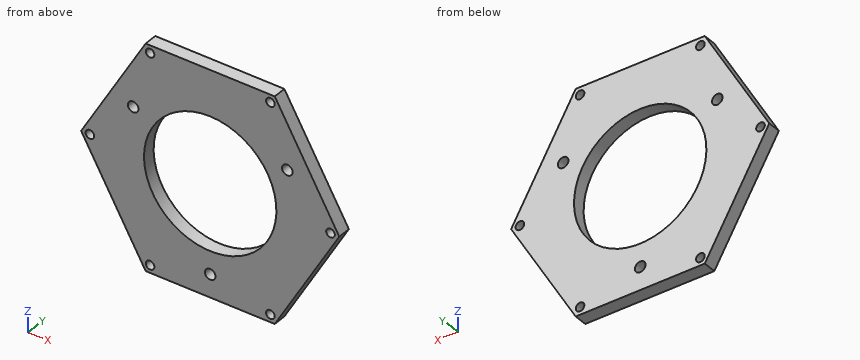
```python
from build123d import *

# Parameters (mm, degrees)
BOSS_EXTRUDE1_DEPTH = 4
SKETCH3_R           = 20
CUT_EXTRUDE1_DEPTH  = 4
SKETCH4_R           = 1.6
SKETCH4_R_2         = 1.3
CUT_EXTRUDE2_DEPTH  = 4


with BuildPart() as part:
    # Sketch2 → Boss-Extrude1 (new body)
    with BuildSketch(Plane(origin=(0, 0, 0), x_dir=(1, 0, 0), z_dir=(0, 1, 0))):
        Polygon((1.572650536, 74.401195204), (-37.427349464, 74.401195204), (-56.927349464, 40.626204456), (-37.427349464, 6.851213708), (1.572650536, 6.851213708), (21.072650536, 40.626204456), align=None)
    extrude(amount=-BOSS_EXTRUDE1_DEPTH)

    # Sketch3 → Cut-Extrude1 (cut)
    with BuildSketch(Plane(origin=(0, 0, 0), x_dir=(1, 0, 0), z_dir=(0, 1, 0))):
        with Locations(Location((-17.927354806, 40.626195204, 0), (0, 0, 270))):
            Circle(SKETCH3_R)
    extrude(amount=-CUT_EXTRUDE1_DEPTH, mode=Mode.SUBTRACT)

    # Sketch4 → Cut-Extrude2 (cut)
    with BuildSketch(Plane(origin=(0, 0, 0), x_dir=(1, 0, 0), z_dir=(0, 1, 0))):
        with Locations(Location((5.360065631, 27.181209082, 0), (0, 0, 270))):
            Circle(SKETCH4_R)
        with Locations(Location((0.244744901, 9.15121368, 0), (0, 0, 270))):
            Circle(SKETCH4_R_2)
        with Locations(Location((-36.099443845, 9.151213708, 0), (0, 0, 270))):
            Circle(SKETCH4_R_2)
        with Locations(Location((-41.214764559, 27.181190577, 0), (0, 0, 270))):
            Circle(SKETCH4_R)
        with Locations(Location((-17.927365489, 67.516185951, 0), (0, 0, 270))):
            Circle(SKETCH4_R)
        with Locations(Location((18.416839298, 40.626204456, 0), (0, 0, 270))):
            Circle(SKETCH4_R_2)
        with Locations(Location((0.244744917, 72.101195204, 0), (0, 0, 270))):
            Circle(SKETCH4_R_2)
        with Locations(Location((-54.271538226, 40.626204456, 0), (0, 0, 270))):
            Circle(SKETCH4_R_2)
        with Locations(Location((-36.099443845, 72.101195204, 0), (0, 0, 270))):
            Circle(SKETCH4_R_2)
    extrude(amount=-CUT_EXTRUDE2_DEPTH, mode=Mode.SUBTRACT)


solid = part.part
```
Read the model definition and answer for the solid it produces. Units are mm, in the model's axes. Round coordinates to 2 decimals unless told otherwise and drop trailing zeros. Write each loop counter-clockwise with the first axis right and the second up, starting at its lowest first coordinate (ties: lowest second). Pieces come first, ordered by that corner, then holes. Notation, with made-up numbers: (-20, -36.5) - (-8, -36.5) arc R19 ccw to (-8, -24.5) - close; hole circle Ø7 at (60, 63). An arc over 180 degrees is marked (long way). One line per item, written item: value.
Q1. Straight lines are drawn through the part: line 1 (X direction, y = -2.5, z = -28.5); line 2 (Z direction, x = -19, y = -1.35); line 3 (Z direction, x = 18, y = -0.8). For each, find the intervals that lie inside material, in ascending order. Write a range as from..to.
The answers:
line 1: x = -49.93..-42.12, -40.31..-33.83, -2.02..4.45, 6.27..14.07
line 2: z = -74.4..-68.7, -66.33..-60.6, -20.65..-6.85
line 3: z = -45.95..-41.86, -39.39..-35.3
Q2. Find section C-C (y = -3.4). Count the separate pieces of the cut face and the enclosed holes in it, and give its area (3 significant figures).
The answers:
separate pieces: 1
enclosed holes: 10
area: 2,640 mm2
Q3. Find section A-A (z = -24). Determine the outline of the cut face in (x, y), and give its area (3 significant figures).
The answers:
outline: (-47.33, -4) - (-29.04, -4) - (-29.04, 0) - (-47.33, 0) - close; (-6.81, -4) - (11.47, -4) - (11.47, 0) - (-6.81, 0) - close
area: 146 mm2
Q4. Find section D-D (x = -50). Determine the outline of the cut face in (y, z).
The answers:
outline: (-4, -52.62) - (0, -52.62) - (0, -28.63) - (-4, -28.63) - close
Q5. This flat-tipped pin is pushed along its axis until it touches: P1, Ø1, axis at y = -1.5, z = -46, coming from the +X side. Where does it stop, or does it pass through?
The answers:
P1: stops at x = 18.26
Q6. Find section B-B (x = -14). Determine the outline of the cut face in (y, z), and give its area (3 significant figures).
The answers:
outline: (-4, -74.4) - (0, -74.4) - (0, -60.24) - (-4, -60.24) - close; (-4, -21.02) - (0, -21.02) - (0, -6.85) - (-4, -6.85) - close
area: 113 mm2
